Check sheet for the modelled part. Datum: model origin and axes. Units: mm. A direction names the side the tool comes from. Coordinates: 2 decimals unless noted, no trailing zeros. Loops run counter-clockwise (first coordinate to the right, second up) from the corner with the lowest first, then second, coordinate; pieces in that order, holes last. Notation, with made-up numbers: (26.5, -31) - (79.5, -31) arc R17 cw to (79.5, -4) - close; hole circle Ø5 at (77, -25.5). An arc over 180 degrees is marked (long way). Use a Markdown table: item, result. Add a question column.
1) Go/stop test with flat-tipped pins: P1, Ø6, axis at x = 55.5, y = -2.5, coming from the +Z side; P2, Ø10, axis at y = 7.5, z = -181, coming from the +X side; P3, Ø5.5, axis at x = 98, y = -1, coming from the -Z side; P4, Ø2, axis at x = -3.18, y = 8.75, coming from the -Z side. Record where each tip stops, or that it passes through.
2) Draft check along X on faces 1 (the flat face through (12.7, 0, -108)), 2 (the flat face through (6.35, 0, -113)), 3 (the flat face through (-3, 0, 0)). Enter one of: pulls with the +X half, pulls with the -X half, needs draft (parallel to the pull), parting line crosses it, or undercut.
3) Sectioned sample at C-C, the plane x = 77. Enter the section's corners in (y, z), then the cut area to 3 significant figures.
4) Thickness scan on line 1 (X direction, y = -9.25, z = -106); line 2 (Z direction, x = 90.5, y = -6.25) (3 decimals); line 3 (Z direction, x = 27, y = 6.5). Record the ranges inside material, lowest first.
5) Sectioned sample at A-A, the plane z = -211.5. Enter the section's corners in (x, y), then the cut area to 3 significant figures.
6) Sectioned sample at B-B, the plane y = -3.5. Enter the section's corners in (x, z) (3 decimals).
7) Tool access check on faces 4 (the flat face through (95, 0, 0)), 5 (the flat face through (46, 0, -228.6)), 6 (the flat face through (46, 0, -222.25)). Record the directions out of +Z, -Z, +X, -X, +Y, -Y that give a thin tool (end or side, any length) a straight path to the whole face; none if there is none.
from build123d import *

# Parameters (mm, degrees)
SKETCH1_W             = 25.4
SKETCH1_H             = 25.4
BOSS_EXTRUDE1_DEPTH   = 3.175
SKETCH3_W             = 6.35
SKETCH3_H             = 25.4
BOSS_EXTRUDE2_DEPTH   = 228.6
F_4_40_TAPPED_HOLE1_D = 2.2606
SKETCH7_W             = 6.35
SKETCH7_H             = 25.4
BOSS_EXTRUDE3_DEPTH   = 73.152
SKETCH9_W             = 6.35
SKETCH9_H             = 25.4
BOSS_EXTRUDE4_DEPTH   = 222.25
SKETCH10_W            = 25.4
SKETCH10_H            = 25.4
BOSS_EXTRUDE5_DEPTH   = 3.175
F_4_40_TAPPED_HOLE4_D = 2.2606
BOSS_EXTRUDE6_START   = -3.175
SKETCH16_R            = 1.1303
BOSS_EXTRUDE6_DEPTH   = 3.175


with BuildPart() as part:
    # Sketch1 → Boss-Extrude1 (new body)
    with BuildSketch(Plane.XY):
        Rectangle(SKETCH1_W, SKETCH1_H)
    extrude(amount=BOSS_EXTRUDE1_DEPTH)

    # Sketch3 → Boss-Extrude2 (add)
    with BuildSketch(Plane(origin=(0, 0, 0), x_dir=(-1, 0, 0), z_dir=(0, 0, -1))):
        with Locations((-9.525, 0)):
            Rectangle(SKETCH3_W, SKETCH3_H)
    extrude(amount=BOSS_EXTRUDE2_DEPTH)

    # #4-40 Tapped Hole1 (through all)
    with Locations(Plane(origin=(0, 0, 0), x_dir=(-1, 0, 0), z_dir=(0, 0, -1))):
        with Locations((3.175, 8.746639232), (3.175, -8.393153768)):
            Hole(F_4_40_TAPPED_HOLE1_D / 2)

    # Sketch7 → Boss-Extrude3 (add)
    with BuildSketch(Plane(origin=(12.7, 0, 0), x_dir=(0, 0, -1), z_dir=(1, 0, 0))):
        with Locations((225.425, 0)):
            Rectangle(SKETCH7_W, SKETCH7_H)
    extrude(amount=BOSS_EXTRUDE3_DEPTH)

    # Sketch9 → Boss-Extrude4 (add)
    with BuildSketch(Plane.XY.offset(-222.25)):
        with Locations((82.677, 0)):
            Rectangle(SKETCH9_W, SKETCH9_H)
    extrude(amount=BOSS_EXTRUDE4_DEPTH)

    # Sketch10 → Boss-Extrude5 (add)
    with BuildSketch(Plane.XY):
        with Locations((92.202, 0)):
            Rectangle(SKETCH10_W, SKETCH10_H)
    extrude(amount=BOSS_EXTRUDE5_DEPTH)

    # #4-40 Tapped Hole4 (through all)
    with Locations(Plane.XY.offset(3.175)):
        with Locations((100.484060812, 7.185260309), (95.382, 8.746639232), (95.382, -8.393153768)):
            Hole(F_4_40_TAPPED_HOLE4_D / 2)

    # Sketch16 → Boss-Extrude6 (add)
    with BuildSketch(Plane.XY.offset(3.175).offset(BOSS_EXTRUDE6_START)):
        with Locations((100.484060812, 7.185260309)):
            Circle(SKETCH16_R)
    extrude(amount=BOSS_EXTRUDE6_DEPTH)


solid = part.part
Solved:
| question | item | result |
|---|---|---|
| 1 | P1 | stops at z = -222.25 |
| 1 | P2 | stops at x = 85.85 |
| 1 | P3 | stops at z = 0 |
| 1 | P4 | passes through |
| 2 | face 1 | undercut |
| 2 | face 2 | pulls with the -X half |
| 2 | face 3 | needs draft |
| 3 | outline | (-12.7, -228.6) - (12.7, -228.6) - (12.7, -222.25) - (-12.7, -222.25) - close |
| 3 | area | 161 mm2 |
| 4 | line 1 | x = 6.35 to 12.7, 79.5 to 85.85 |
| 4 | line 2 | z = 0 to 3.175 |
| 4 | line 3 | z = -228.6 to -222.25 |
| 5 | outline | (6.35, -12.7) - (12.7, -12.7) - (12.7, 12.7) - (6.35, 12.7) - close; (79.5, -12.7) - (85.85, -12.7) - (85.85, 12.7) - (79.5, 12.7) - close |
| 5 | area | 323 mm2 |
| 6 | outline | (-12.7, 0) - (6.35, 0) - (6.35, -228.6) - (85.852, -228.6) - (85.852, 0) - (104.902, 0) - (104.902, 3.175) - (79.502, 3.175) - (79.502, -222.25) - (12.7, -222.25) - (12.7, 3.175) - (-12.7, 3.175) - close |
| 7 | face 4 | -Z, +X, +Y, -Y |
| 7 | face 5 | -Z, +X, -X, +Y, -Y |
| 7 | face 6 | +Z, +Y, -Y |
